The model under review builds one solid part; all positions refer to its coordinate system, in mm. A direction names the side the tool comes from. Coordinates: 2 decimals unless noted, no trailing zeros. Write each loop counter-clockwise with the first axis right and the second up, starting at its lowest first coordinate (ties: lowest second). Pieces come first, ordered by that corner, then holes. Notation, with made-up numbers: (-16, -3.5) - (13, -3.5) arc R27 ccw to (13, 31.5) - close; hole circle Ø6 at (16.25, 82.5). An arc over 180 degrees is marked (long way). Put each result on its own line as item: value.
Autodesk Inventor part; units mm, degrees
ref_plane "Work Plane1" through (6.25, 0, 0) normal (1, 0, 0) x (0, 0, -1)
ref_plane "YZ Plane" through (0, 0, 0) normal (1, 0, 0) x (0, 1, 0)
ref_plane "XZ Plane" through (0, 0, 0) normal (0, 1, 0) x (-1, 0, 0)
sketch "Sketch1" plane through (0, 0, 0) normal (0, 0, 1) x (1, 0, 0)
  line L0 (0, 0) -> (12.5, 0)
  line L1 (12.5, 0) -> (12.5, 14.5)
  line L2 (12.5, 14.5) -> (0, 14.5)
  line L3 (0, 14.5) -> (0, 0)
  dimension "d0" = 14.5
  dimension "d1" = 12.5
extrude "Extrusion1" add sketch "Sketch1" against normal blind 18.5
sketch "Sketch2" plane through (0, 0, -18.5) normal (0, 0, -1) x (-1, 0, 0)
  circle A0 centre (-9.9, 3.6) radius 2.5
  circle A1 centre (-2.6, 3.6) radius 2.5
  circle A2 centre (-2.6, 10.9) radius 2.5
  circle A3 centre (-9.9, 10.9) radius 2.5
  line L0 (-9.9, 10.9) -> (-9.9, 3.6) construction
  line L1 (-12.5, 14.5) -> (-12.5, 0) construction
  line L2 (-9.9, 10.9) -> (-2.6, 10.9) construction
  line L3 (0, 14.5) -> (-12.5, 14.5) construction
  line L4 (-7.4, 10.9) -> (-5.1, 10.9)
  line L5 (-2.6, 8.4) -> (-2.6, 6.1)
  line L6 (-7.4, 3.6) -> (-5.1, 3.6)
  line L7 (-9.9, 8.4) -> (-9.9, 6.1)
  circle A4 centre (-9.9, 10.9) radius 1.75
  circle A5 centre (-2.6, 10.9) radius 1.75
  circle A6 centre (-2.6, 3.6) radius 1.75
  circle A7 centre (-9.9, 3.6) radius 1.75
  circle A8 centre (-6.25, 7.25) radius 1.57
  point P0 (0, 0)
  point P1 (-9.9, 7.25)
  point P2 (-12.5, 7.25)
  point P3 (-6.25, 10.9)
  point P4 (-6.25, 14.5)
  point P5 (-6.25, 3.6)
  point P6 (-2.6, 7.25)
  dimension "d4" = 5
  dimension "d5" = 12.3
  dimension "d6" = 7.3
  dimension "d7" = 0.75
  dimension "d8" = 3.14
sketch "Sketch3" plane through (0, 0, 0) normal (0, 0, 1) x (1, 0, 0)
  circle A0 centre (6.25, 7.1995) radius 1.65
  point P0 (0, 0)
  dimension "d9" = 3.3
extrude "Extrusion2" add sketch "Sketch3" along normal blind 5
extrude "Extrusion3" add sketch "Sketch2" along normal blind 6.52
extrude "Extrusion4" add sketch "Sketch2" along normal blind 12.52 contours A8
ref_plane "Work Plane1" through (6.25, 0, 0) normal (1, 0, 0) x (0, 0, -1)
sketch "Sketch4" plane through (6.25, 0, 0) normal (1, 0, 0) x (0, 0, -1)
  line L0 (18.5, 10.9) -> (25.02, 10.9)
  line L1 (21.76, 10.9) -> (23.385, 10.9)
  line L2 (23.385, 10.9) -> (23.385, 14.1)
  line L3 (23.385, 18.1) -> (21.76, 18.1)
  line L4 (21.76, 18.1) -> (21.76, 10.9)
  line L5 (21.76, 10.9) -> (23.385, 10.9)
  line L6 (23.385, 10.9) -> (23.385, 14.1)
  line L7 (21.76, 18.1) -> (21.76, 15.1)
  line L8 (23.6683, 15.1) -> (23.81, 15.1)
  line L9 (23.81, 15.1) -> (23.385, 18.1)
  line L10 (21.76, 18.1) -> (21.76, 14.1)
  line L11 (23.385, 14.1) -> (23.81, 14.1)
  line L12 (23.81, 14.1) -> (23.6683, 15.1)
  point P0 (0, 0)
  dimension "d16" = 1.625
  dimension "d17" = 7.2
  dimension "d18" = 90
  dimension "d19" = 3
  dimension "d20" = 2.05
  dimension "d21" = 4
  dimension "d22" = 1.625
  dimension "d23" = 2.05
  dimension "d24" = 3
revolve "Revolution1" add sketch "Sketch4" angle 360 about axis through (6.25, 18.1, -21.76) along (0, -1, 0)
pattern_circular "Circular Pattern1" count 4 over 360 about axis through (6.25, 7.25, -18.5) along (0, 0, -1) of "Revolution1"
delete faces "Delete Face1" heal yes whole lump no faces at (8.0785, 15.7667, -22.4534) (5.7435, 18.1, -22.5272) (8.079, 14.2111, -22.6505) (7.3088, 12.1519, -20.5273) (6.0865, 14.1, -23.6485) (6.0865, 15.1, -23.7429) (14.7667, 7.718, -23.6587) (14.1, 6.0575, -23.3527) (13.2111, 5.421, -22.6505) (13.1, 7.4135, -23.6485) (11.1519, 6.1912, -20.5273) (17.1, 7.7565, -22.5272) (6.718, -1.2667, -23.6587) (4.421, 0.2889, -22.6505) (5.0575, -0.6, -23.3527) (6.4135, 0.4, -23.6485) (5.1912, 2.3481, -20.5273) (6.7565, -3.6, -22.5272)
properties part number "Adafruit_1528-4663-ND"
1. To check wall thickness, follow probe 1 along Y at (x, z) = (2.6, -22.5); probe 2 along X at (y, z) = (2.25, -19); probe 3 along X at (y, z) = (9.75, -24.5). State the ranges of each line that lie inside material, in increasing order.
Determined:
probe 1: y = 1.1 to 1.85, 5.35 to 9.15, 12.65 to 13.4
probe 2: x = 0.5 to 1.49, 3.71 to 4.7, 7.8 to 8.79, 11.01 to 12
probe 3: x = 0.38 to 1.28, 3.92 to 8.58, 11.22 to 12.12
2. Machinability: for faces 1 (the cylindrical face through (2.98, 12.61, -21.71)), 2 (the cylindrical face through (5.034, 6.084, 2.465)), 3 (the flat face through (12.5, 7, -9)), 4 (the cylindrical face through (0.622, 7.179, -20.137)), 5 (the flat face through (9.9, 7, -22)), which of the approach directions +Z, -Z, +X, -X, +Y, -Y give a long, thin tool a straight path to every point of the face, cutting with its end or side? Answer none if there is none.
Determined:
face 1: -Z
face 2: +Z
face 3: +Z, -Z, +X, +Y, -Y
face 4: none
face 5: -Z, +X
3. Consider section A-A on x = 1.25. State the section outline as (y, z) points (3 decimals).
Determined:
outline: (0, -18.5) - (1.496, -18.5) - (1.496, -25.02) - (2.486, -25.02) - (2.486, -18.5) - (4.714, -18.5) - (4.714, -25.02) - (5.704, -25.02) - (5.704, -22.261) arc R1.625 ccw to (8.796, -22.261) - (8.796, -25.02) - (9.786, -25.02) - (9.786, -18.5) - (12.014, -18.5) - (12.014, -25.02) - (13.004, -25.02) - (13.004, -18.5) - (14.5, -18.5) - (14.5, 0) - (0, 0) - close; hole (5.704, -21.259) arc R1.625 cw to (8.796, -21.259) - (8.796, -18.5) - (5.704, -18.5) - close
4. Consider section B-B on z = -21.76. State the section outline as (x, y) points (3 decimals).
Determined:
outline: (-4.6, 5.625) - (-1.6, 5.2) - (-1.6, 5.342) - (-0.6, 5.2) - (-0.6, 5.625) - (1.134, 5.625) arc R2.5 ccw (long way) to (5.1, 3.6) - (7.4, 3.6) arc R2.5 ccw (long way) to (9.9, 6.1) - (9.9, 8.4) arc R2.5 ccw (long way) to (7.4, 10.9) - (5.1, 10.9) arc R2.5 ccw (long way) to (1.134, 8.875) - (-0.6, 8.875) - (-0.6, 9.3) - (-1.6, 9.158) - (-1.6, 9.3) - (-4.6, 8.875) - close; hole circle Ø3.5 at (2.6, 3.6); hole circle Ø3.5 at (2.6, 10.9); hole circle Ø3.5 at (9.9, 3.6); hole circle Ø3.5 at (9.9, 10.9)
5. The part is to be moulded in two halves that separate along X. For faces 6 (the flat face through (5, 6, -25.02)), 7 (the cylindrical face through (7.5, 8.2, -28)), 8 (the flat face through (10, 4, -18.5)), say which applies: +X half, -X half, draft (parallel to the pull), parting line (faces both ways), or undercut.
Determined:
face 6: draft
face 7: parting line
face 8: undercut
6. Consider section D-D on z = -27. State the section outline as (x, y) points, plus the area to 3 significant figures.
Determined:
outline: circle Ø3.14 at (6.25, 7.25)
area: 7.74 mm^2
7. Consider section C-C on y = 4.75. State the section outline as (x, z) points.
Determined:
outline: (0, -18.5) - (0.38, -18.5) - (0.38, -25.02) - (1.28, -25.02) - (1.28, -18.5) - (3.92, -18.5) - (3.92, -25.02) - (8.58, -25.02) - (8.58, -18.5) - (11.22, -18.5) - (11.22, -25.02) - (12.12, -25.02) - (12.12, -18.5) - (12.5, -18.5) - (12.5, 0) - (0, 0) - close
8. For pin 1 Ø0.7 at (x, z) = (6, -21) entering from -Y; pin 2 Ø3 at (x, y) = (2.6, 3.6) entering from +Z; pin 3 Ø2.5 at (y, z) = (6.5, -20.5) entering from +X, all flat-tipped, find the tip position at first contact; note any pin that passes through.
Determined:
pin 1: stops at y = 3.6
pin 2: stops at z = 0
pin 3: stops at x = 11.78
